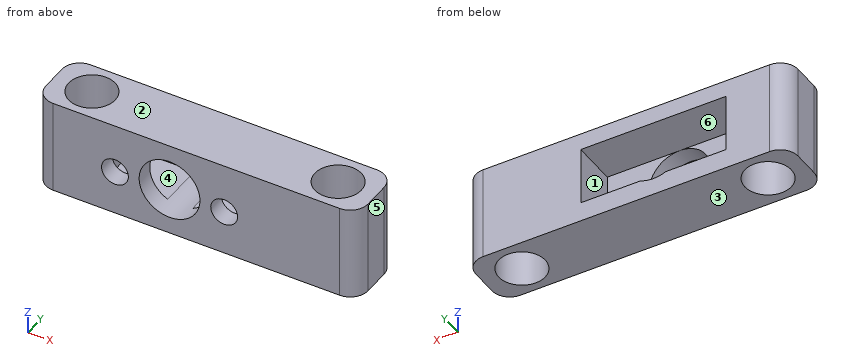
```python
from build123d import *

# Parameters (mm, degrees)
CROQUIS1_W              = 36
CROQUIS1_H              = 7
CROQUIS1_R              = 2.6
SALIENTE_EXTRUIR1_DEPTH = 10.6
CROQUIS5_R              = 3.4
CORTAR_EXTRUIR4_DEPTH   = 7
REDONDEO1_R             = 2
CROQUIS7_W              = 16.2
CROQUIS7_H              = 6.4
CORTAR_EXTRUIR5_DEPTH   = 5
CROQUIS8_R              = 1.5
CORTAR_EXTRUIR6_DEPTH   = 2
CROQUIS9_W              = 16.2
CROQUIS9_H              = 6.2
CORTAR_EXTRUIR7_DEPTH   = 5


with BuildPart() as part:
    # Croquis1 → Saliente-Extruir1 (new body)
    with BuildSketch(Plane.XY):
        with Locations((-28.016694491, 12.37804878)):
            Rectangle(CROQUIS1_W, CROQUIS1_H)
        with Locations((-41.766694491, 12.37804878)):
            Circle(CROQUIS1_R, mode=Mode.SUBTRACT)
        with Locations((-14.266694491, 12.37804878)):
            Circle(CROQUIS1_R, mode=Mode.SUBTRACT)
    extrude(amount=SALIENTE_EXTRUIR1_DEPTH)

    # Croquis5 → Cortar-Extruir4 (cut)
    with BuildSketch(Plane.XZ.offset(-8.87804878)):
        with Locations(Location((-31.016694491, 5.3, 0), (0, 0, 270))):
            Circle(CROQUIS5_R)
    extrude(amount=-CORTAR_EXTRUIR4_DEPTH, mode=Mode.SUBTRACT)

    # Redondeo1
    redondeo1_edges = [part.edges().sort_by_distance(p)[0] for p in [
        (-46.016694491, 15.87804878, 5.3),
        (-10.016694491, 15.87804878, 5.3),
        (-10.016694491, 8.87804878, 5.3),
        (-46.016694491, 8.87804878, 5.3),
    ]]
    fillet(redondeo1_edges, radius=REDONDEO1_R)

    # Croquis7 → Cortar-Extruir5 (cut)
    with BuildSketch(Plane(origin=(0, 15.87804878, 0), x_dir=(1, 0, 0), z_dir=(0, 1, 0))):
        with Locations((-31.016694491, -5.5)):
            Rectangle(CROQUIS7_W, CROQUIS7_H)
    extrude(amount=-CORTAR_EXTRUIR5_DEPTH, mode=Mode.SUBTRACT)

    # Croquis8 → Cortar-Extruir6 (cut)
    with BuildSketch(Plane(origin=(0, 10.87804878, 0), x_dir=(1, 0, 0), z_dir=(0, 1, 0))):
        with Locations(Location((-24.916694491, -5, 0), (0, 0, 270))):
            Circle(CROQUIS8_R)
        with Locations(Location((-37.116694491, -5, 0), (0, 0, 270))):
            Circle(CROQUIS8_R)
    extrude(amount=-CORTAR_EXTRUIR6_DEPTH, mode=Mode.SUBTRACT)

    # Croquis9 → Cortar-Extruir7 (cut)
    with BuildSketch(Plane(origin=(0, 15.87804878, 0), x_dir=(1, 0, 0), z_dir=(0, 1, 0))):
        with Locations((-31.016694491, -5.3)):
            Rectangle(CROQUIS9_W, CROQUIS9_H)
    extrude(amount=-CORTAR_EXTRUIR7_DEPTH, mode=Mode.SUBTRACT)


solid = part.part
```
Read the model definition and answer for the solid it produces. Units are mm, in the model's axes. Face numbers are marked on the shaded views. A direction names the side the tool comes from. Give positions to 0.01 mm unless a question says otherwise; leave off trailing zeros. Write each loop counter-clockwise with the first axis right and the second up, starting at its lowest first coordinate (ties: lowest second). Pieces come first, ordered by that corner, then holes. Notation, with made-up numbers: M 14,26.25 L 43,26.25 A20 ccw 43,39.25 Z; hole C -5,70.5 d8. An arc over 180 degrees is marked long. Put each result on its own line as item: value. Start each with the question number.
1. For a pull along Z with two mould halves and no side action, classify the marked faces 3, 4, 5 and 6 as released by +Z, released by -Z, zero draft, split by the parting line, or undercut.
2. The part is cut by section C-C, the plane x = -24.5. Give the vertices of the cut face in (y, z), and give its area (3 significant figures).
3. The part is cut by section D-D, the plane x = -14. Give the vertices of the cut face in (y, z).
4. The part is cut by section B-B, the plane y = 13.5. Give the vertices of the cut face in (x, z).
5. Which of the six approach directions +Z, -Z, +X, -X, +Y, -Y give full straight-line access (tool end or side, diameter ignored) to the marked faces 1 and 2?
6. Consider line 1 along Z through (x, y) = (-36, 14.5); line 2 along X through (y, z) = (14, 7); line 3 along X through (y, z) = (9.5, 6). Determine where each line is inside the solid, lowest interval first.
7. Each of these flat-tipped pins is pushed along its axis until it touches: pin 1 Ø5.5 at (x, z) = (-31.02, 5.3) entering from +Y; pin 2 Ø3 at (x, z) = (-34.5, 6.5) entering from +Y. Where does it stop, or does it pass through?
8. The part is cut by section A-A, the plane z = 5. Give the vertices of the cut face in (x, y).
Final values:
1. face 3: released by -Z
1. face 4: undercut
1. face 5: zero draft
1. face 6: undercut
2. outline: M 8.88,0 L 15.88,0 L 15.88,2.2 L 10.88,2.2 L 10.88,3.56 L 8.88,3.56 Z; M 8.88,6.44 L 10.88,6.44 L 10.88,8.7 L 15.88,8.7 L 15.88,10.6 L 8.88,10.6 Z
2. area: 35.9 mm²
3. outline: M 8.88,0 L 9.79,0 L 9.79,10.6 L 8.88,10.6 Z; M 14.96,0 L 15.88,0 L 15.88,10.6 L 14.96,10.6 Z
4. outline: M -46.02,0 L -44.11,0 L -44.11,10.6 L -46.02,10.6 Z; M -39.42,0 L -16.61,0 L -16.61,10.6 L -39.42,10.6 Z; M -11.92,0 L -10.02,0 L -10.02,10.6 L -11.92,10.6 Z; hole M -39.12,2.2 L -32.41,2.2 A3.4 ccw -29.62,2.2 L -22.92,2.2 L -22.92,8.7 L -39.12,8.7 Z
5. face 1: +Y
5. face 2: +Z, +X, -X, +Y, -Y
6. line 1: z = 0 to 2.2, 8.7 to 10.6
6. line 2: x = -46.01 to -43.8, -39.73 to -39.12, -22.92 to -16.3, -12.23 to -10.02
6. line 3: x = -45.47 to -38.23, -36 to -34.34, -27.69 to -26.03, -23.8 to -10.57
7. pin 1: passes through
7. pin 2: stops at y = 10.88
8. outline: M -46.02,10.88 A2 ccw -44.02,8.88 L -38.62,8.88 L -38.62,10.88 L -39.12,10.88 L -39.12,15.88 L -44.02,15.88 A2 ccw -46.02,13.88 Z; M -35.62,8.88 L -34.4,8.88 L -34.4,10.88 L -35.62,10.88 Z; M -27.63,8.88 L -26.42,8.88 L -26.42,10.88 L -27.63,10.88 Z; M -23.42,8.88 L -12.02,8.88 A2 ccw -10.02,10.88 L -10.02,13.88 A2 ccw -12.02,15.88 L -22.92,15.88 L -22.92,10.88 L -23.42,10.88 Z; hole C -41.77,12.38 d5.2; hole C -14.27,12.38 d5.2
